```python
from build123d import *

# Parameters (mm, degrees)
BOSS_EXTRUDE3_START = -7.103375673
SKETCH4_R           = 2.125
SKETCH4_R_2         = 4.25
BOSS_EXTRUDE3_DEPTH = 7.103375673
BOSS_EXTRUDE4_START = 5
SKETCH6_R           = 8
SKETCH6_R_2         = 2.125
BOSS_EXTRUDE4_DEPTH = 5
SKETCH5_R           = 4
CUT_EXTRUDE2_DEPTH  = 9.103375673
CHAMFER2_SIZE       = 1.154700538
CHAMFER2_SIZE_2     = 2
CHAMFER3_SIZE       = 3


# Read off the part's stored shape, not the designer's step: Revolve1
with BuildPart() as part:
    # Revolve1 outline → Revolve1 (revolve)
    with BuildSketch(Plane.XY):
        Polygon((4.25, 0), (3.8, -0.45), (3.55, -0.45), (3.55, -2.56), (2, -2.56), (2, -1.7), (0.8, -0.5), (0.5, -0.5), (0.5, -3.56), (3, -5.003375673), (3, -6.353375673), (2, -6.353375673), (3.299038106, -7.103375673), (4.25, -7.103375673), align=None)
    revolve(axis=Axis((0, 0, 0), (0, 1, 0)))

    # Sketch4 → Boss-Extrude3 (add)
    with BuildSketch(Plane.XZ.offset(7.103375673).offset(BOSS_EXTRUDE3_START)):
        with BuildLine():
            Line((-7, 4.875), (7, 4.875))
            Line((7, 4.875), (8.680016564, 6.228945842))
            ThreePointArc((8.680016564, 6.228945842), (21.7, 0), (8.680016564, -6.228945842))
            Line((8.680016564, -6.228945842), (7, -4.875))
            Line((7, -4.875), (-7, -4.875))
            Line((-7, -4.875), (-8.680016564, -6.228945842))
            ThreePointArc((-8.680016564, -6.228945842), (-21.7, 0), (-8.680016564, 6.228945842))
            Line((-8.680016564, 6.228945842), (-7, 4.875))
        make_face()
        with Locations(Location((-13.7, 0, 0), (0, 0, 270))):
            Circle(SKETCH4_R, mode=Mode.SUBTRACT)
        with Locations(Location((13.7, 0, 0), (0, 0, 270))):
            Circle(SKETCH4_R, mode=Mode.SUBTRACT)
        Circle(SKETCH4_R_2, mode=Mode.SUBTRACT)
    extrude(amount=BOSS_EXTRUDE3_DEPTH)

    # Sketch6 → Boss-Extrude4 (add)
    # profile 1 of 2: a face of its own
    with BuildSketch(Plane(origin=(0, 0, 0), x_dir=(1, 0, 0), z_dir=(0, 1, 0)).offset(BOSS_EXTRUDE4_START)):
        with Locations(Location((-13.7, 0, 0), (0, 0, 51.134235394))):
            Circle(SKETCH6_R)
        with Locations(Location((-13.7, 0, 0), (0, 0, 90))):
            Circle(SKETCH6_R_2, mode=Mode.SUBTRACT)
    # profile 2 of 2: a face of its own
    with BuildSketch(Plane(origin=(0, 0, 0), x_dir=(1, 0, 0), z_dir=(0, 1, 0)).offset(BOSS_EXTRUDE4_START)):
        with Locations(Location((13.7, 0, 0), (0, 0, 128.865764606))):
            Circle(SKETCH6_R)
        with Locations(Location((13.7, 0, 0), (0, 0, 90))):
            Circle(SKETCH6_R_2, mode=Mode.SUBTRACT)
    extrude(amount=-BOSS_EXTRUDE4_DEPTH)

    # Sketch5 → Cut-Extrude2 (cut)
    with BuildSketch(Plane.XZ.offset(7.103375673)):
        with Locations(Location((-13.699999648, 0, 0), (0, 0, 270))):
            Circle(SKETCH5_R)
        with Locations(Location((13.7, 0, 0), (0, 0, 270))):
            Circle(SKETCH5_R)
    extrude(amount=-CUT_EXTRUDE2_DEPTH, mode=Mode.SUBTRACT)

    # Chamfer2
    # the kernel refuses this chamfer: 2, 1.154700538 mm, written as the material it adds along each edge
    with BuildSketch(Plane(origin=(-13.699999648, 2, 0), x_dir=(0, 0, -1), z_dir=(-1, 0, 0))) as chamfer2_piece_1_section:
        Polygon((4, CHAMFER2_SIZE), (4 - CHAMFER2_SIZE_2, 0), (4, 0), align=None)
    chamfer2_piece_1 = revolve(axis=Axis((-13.699999648, 2, 0), (0, -1, 0)), mode=Mode.PRIVATE)
    chamfer2_piece_1 = chamfer2_piece_1 - Plane(origin=(-13.7, 1.411589212, 0), x_dir=(0, 0, -1), z_dir=(0, 1, 0)) * Cylinder(2.125, 17, mode=Mode.PRIVATE)
    add(chamfer2_piece_1)
    with BuildSketch(Plane(origin=(13.7, 2, 0), x_dir=(0, 0, -1), z_dir=(-1, 0, 0))) as chamfer2_piece_2_section:
        Polygon((4, CHAMFER2_SIZE), (4 - CHAMFER2_SIZE_2, 0), (4, 0), align=None)
    chamfer2_piece_2 = revolve(axis=Axis((13.7, 2, 0), (0, -1, 0)), mode=Mode.PRIVATE)
    chamfer2_piece_2 = chamfer2_piece_2 - Plane(origin=(13.7, 1.41158911, 0), x_dir=(0, 0, -1), z_dir=(0, 1, 0)) * Cylinder(2.125, 16, mode=Mode.PRIVATE)
    add(chamfer2_piece_2)

    # Chamfer3
    chamfer3_edges = [part.edges().sort_by_distance(p)[0] for p in [
        (-18.719983436, 5, 6.228945842),
        (18.719983436, 5, 6.228945842),
    ]]
    chamfer(chamfer3_edges, length=CHAMFER3_SIZE)


solid = part.part
```
Source: CAD feature listing. Evaluate the final solid. Frame: model axes, mm. A direction names the side the tool comes from. Give positions to 0.01 mm unless a question says otherwise; leave off trailing zeros. Write each loop counter-clockwise with the first axis right and the second up, starting at its lowest first coordinate (ties: lowest second). Pieces come first, ordered by that corner, then holes. Notation, with made-up numbers: (32, 22.25) - (47, 22.25) arc R18 cw to (47, 40.25) - close; hole circle Ø2 at (79.5, 63.5). An arc over 180 degrees is marked (long way). One line per item, written item: value. Start each with the question number.
Q1. First-contact query: pin 1 Ø4 at (x, z) = (-4, -6.5) entering from +Y; pin 2 Ø7 at (x, z) = (0, 0) entering from +Y; pin 3 Ø4.5 at (x, z) = (0, 0) entering from -Y. Flat tips, straight axial feed; report the tip coordinate or a pass-through.
Q2. Section query B-B, the plane y = -3. Return the cut outline in (x, z) (3 decimals).
Q3. Material intervals for probe 1 along Z at (x, y) = (0, -5.7) (3 decimals); probe 2 along X at (y, z) = (2.8, 0) (3 decimals); probe 3 along X at (y, z) = (3.2, 0) (3 decimals), sorted ascending. Write a range as from..to.
Q4. Draft query along Z for faces 5 (the face through (0, -4, -4.875)), 6 (the face through (2, -2.56, 2)), 7 (the face through (-3, -6, 0)), 8 (the face through (-10.5, 4.8, 4.1)). Return one class per face: +Z half, -Z half, draft (parallel to the pull), parting line (faces both ways), or undercut.
Q5. Set-up query: faces 1 (the face through (-7.828, -3.502, -5.542)), 2 (the face through (-7.9, -3.5, 5.6)), 3 (the face through (15.774, 3.485, 0.461)), 4 (the face through (0.626, -3.65, -0.197)). Return all of +Z, -Z, +X, -X, +Y, -Y with unobstructed straight access to the full face (end or side cutting, diameter ignored); none if empty.
Q6. Section query D-D, the plane y = 2.75. Return the cut outline in (x, z) (3 decimals).
Q7. Section query C-C, the plane x = 13.7. Return the cut outline in (y, z) (3 decimals).
Answer:
1. pin 1: stops at y = 0
1. pin 2: stops at y = -0.5
1. pin 3: stops at y = -6.5
2. outline: (-8.68, -6.229) - (-7, -4.875) - (7, -4.875) - (8.68, -6.229) arc R8 ccw (long way) to (8.68, 6.229) - (7, 4.875) - (-7, 4.875) - (-8.68, 6.229) arc R8 ccw (long way) to start; hole circle Ø8 at (-13.7, 0); hole circle Ø1 at (0, 0); hole circle Ø8 at (13.7, 0)
3. probe 1: z = -4.875..-3, 3..4.875
3. probe 2: x = -20.9..-15.825, -11.575..-6.5, 6.5..11.575, 15.825..20.9
3. probe 3: x = -20.5..-15.825, -11.575..-6.9, 6.9..11.575, 15.825..20.5
4. face 5: -Z half
4. face 6: undercut
4. face 7: undercut
4. face 8: parting line
5. face 1: -Z, +Y, -Y
5. face 2: +Z, +Y, -Y
5. face 3: +Y, -Y
5. face 4: none
6. outline: circle Ø14.5 at (-13.7, 0); circle Ø14.5 at (13.7, 0); hole circle Ø4.25 at (-13.7, 0); hole circle Ø4.25 at (13.7, 0)
7. outline: (-7.103, -8) - (2, -8) - (5, -5) - (5, -2.125) - (1.928, -2.125) - (0.845, -4) - (-7.103, -4) - close; (-7.103, 4) - (0.845, 4) - (1.928, 2.125) - (5, 2.125) - (5, 5) - (2, 8) - (-7.103, 8) - close
